from build123d import *

# Parameters (mm, degrees)
SKETCH2_W           = 12
SKETCH2_H           = 10
BOSS_EXTRUDE1_DEPTH = 3
FILLET1_R           = 1


with BuildPart() as part:
    # Sketch2 → Boss-Extrude1 (new body)
    with BuildSketch(Plane.XY):
        Rectangle(SKETCH2_W, SKETCH2_H)
    extrude(amount=BOSS_EXTRUDE1_DEPTH)

    # Sketch3 → Revolve1 (revolve)
    with BuildSketch(Plane(origin=(0, 0, 0), x_dir=(0, 0, -1), z_dir=(1, 0, 0))):
        Polygon((-3, 0), (-3, 3), (-7, 3), (-7, 2.5), (-12, 2.5), (-12, 0), align=None)
    revolve(axis=Axis((0, 0, 12), (0, 0, -1)))

    # Fillet1
    fillet1_edges = [part.edges().sort_by_distance(p)[0] for p in [
        (-6, 0, 3),
        (6, 0, 3),
    ]]
    fillet(fillet1_edges, radius=FILLET1_R)


solid = part.part
Design review of the part built by this model. Coordinates are the model's own, in mm. A direction names the side the tool comes from. Round coordinates to 2 decimals unless told otherwise and drop trailing zeros. Order: outer loops, then holes, each group sorted by start corner. A loop starts at its lowest first (then second) coordinate and runs counter-clockwise, first axis right, second up.
1) Machinability: for faces 1 (the flat face through (0, 0, 0)), 2 (the cylindrical face through (0, -3, 5)), which of the approach directions +Z, -Z, +X, -X, +Y, -Y give a long, thin tool a straight path to every point of the face, cutting with its end or side? Answer none if there is none.
The answers:
face 1: -Z, +X, -X, +Y, -Y
face 2: +Z
2) For L1, parallel to Z at x = 5, y = 4; L2, parallel to Z at x = 5.75, y = -3.5; L3, parallel to X at y = -2.25, z = 4.75, list the stretches that pass through material, from the lowest coordinate up.
The answers:
L1: z = 0 to 3
L2: z = 0 to 2.66
L3: x = -1.98 to 1.98
3) Clearance check with flat-ended pins moving along their axes: pin 1 Ø5 at (x, y) = (-1, 1) entering from -Z; pin 2 Ø4 at (y, z) = (-2.5, 6.5) entering from +X; pin 3 Ø2 at (x, y) = (-4.5, -1.5) entering from +Z; pin 4 Ø4 at (x, z) = (0, 6) entering from -Y. State where each tip first meets the part, or that it passes through.
The answers:
pin 1: stops at z = 0
pin 2: stops at x = 2.96
pin 3: stops at z = 3
pin 4: stops at y = -3
4) Consider section C-C (x = 4.5). State the section outline as (y, z) points.
The answers:
outline: (-5, 0) - (5, 0) - (5, 3) - (-5, 3) - close
5) Consider section B-B (z = 6.75). State the section outline as (x, y) points, plus the area to 3 significant figures.
The answers:
outline: circle Ø6 at (0, 0)
area: 28.3 mm2
6) Consider section A-A (y = 0). State the section outline as (x, z) points, plus the area to 3 significant figures.
The answers:
outline: (-6, 0) - (6, 0) - (6, 2) arc R1 ccw to (5, 3) - (3, 3) - (3, 7) - (2.5, 7) - (2.5, 12) - (-2.5, 12) - (-2.5, 7) - (-3, 7) - (-3, 3) - (-5, 3) arc R1 ccw to (-6, 2) - close
area: 84.6 mm2
7) Consider section D-D (y = -3.75). State the section outline as (x, z) points.
The answers:
outline: (-6, 0) - (6, 0) - (6, 2) arc R1 ccw to (5, 3) - (-5, 3) arc R1 ccw to (-6, 2) - close
